The listing builds one solid part. Answer for the finished solid, in the listing's coordinates (mm). Give positions to 0.01 mm unless a question says otherwise; leave off trailing zeros. Write each loop counter-clockwise with the first axis right and the second up, starting at its lowest first coordinate (ties: lowest second). Pieces come first, ordered by that corner, then holes. Notation, with made-up numbers: (-24.75, 16) -> (15.25, 16) arc R20 ccw to (15.25, 21) -> close; hole circle Ø5 at (21, 46.5). An arc over 180 degrees is marked (long way). Put each result on its own line as item: value. Start each with the question number.
1) A cutting plane is placed at D-D (y = -71.5). Write down the section's boundary in (x, z), then the cut area to 3 significant figures.
2) A cutting plane is placed at A-A (z = 3.4). Give the number of separate pieces and of enclosed holes in the cut face, then the cut area to 3 significant figures.
3) Find the intervals of material crossed by line 1 along Y through (x, z) = (75, 1.3); line 2 along X through (y, z) = (-91.5, 3.5); line 3 along Y through (x, z) = (89, 3.25), in increasing order. Write a range as from..to.
4) Flat-ended cylindrical pins translate along their axes: pin 1 Ø1.3 at (y, z) = (-39.5, 1.5) entering from +X; pin 2 Ø1.3 at (x, z) = (155.5, 3.5) entering from +Y. Find the tip coordinate at first contact, or state that the pin passes through.
5) A cutting plane is placed at C-C (x = 32.5). Write down the section's boundary in (y, z).
6) A cutting plane is placed at B-B (y = -50). Write down the section's boundary in (x, z), then the cut area to 3 significant figures.
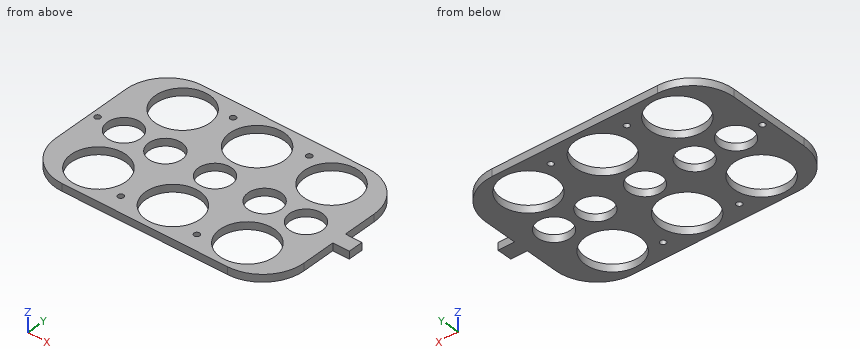
Autodesk Inventor part; units mm, degrees
ref_plane "YZ Plane" through (0, 0, 0) normal (1, 0, 0) x (0, 1, 0)
ref_plane "XZ Plane" through (0, 0, 0) normal (0, 1, 0) x (-1, 0, 0)
ref_plane "XY Plane" through (0, 0, 0) normal (0, 0, 1) x (1, 0, 0)
sketch "Sketch1" plane through (0, 0, 0) normal (0, 0, 1) x (1, 0, 0)
  line L0 (0, 0) -> (150, 0)
  line L1 (150, 0) -> (150, -100)
  line L2 (150, -100) -> (0, -100)
  line L3 (0, -100) -> (0, 0)
  circle A0 centre (30, -20) radius 16.5
  circle A1 centre (30, -80) radius 16.5
  circle A2 centre (75, -20) radius 16.5
  circle A3 centre (120, -20) radius 16.5
  circle A4 centre (75, -80) radius 16.5
  circle A5 centre (120, -80) radius 16.5
  circle A6 centre (20, -50) radius 10
  circle A7 centre (45, -50) radius 10
  circle A8 centre (75, -50) radius 10
  circle A9 centre (105, -50) radius 10
  circle A10 centre (130, -50) radius 10
  circle A11 centre (52, -10) radius 1.75
  circle A12 centre (98, -10) radius 1.75
  circle A13 centre (52, -90) radius 1.75
  circle A14 centre (98, -90) radius 1.75
  circle A15 centre (4, -50) radius 1.75
  dimension "d0" = 150
  dimension "d1" = 100
  dimension "d2" = 33
  dimension "d3" = 33
  dimension "d5" = 33
  dimension "d6" = 33
  dimension "d8" = 33
  dimension "d9" = 33
  dimension "d10" = 20
  dimension "d11" = 20
  dimension "d12" = 20
  dimension "d13" = 30
  dimension "d14" = 30
  dimension "d15" = 75
  dimension "d16" = 30
  dimension "d17" = 75
  dimension "d18" = 30
  dimension "d19" = 20
  dimension "d20" = 20
  dimension "d21" = 20
  dimension "d22" = 20
  dimension "d23" = 20
  dimension "d25" = 20
  dimension "d26" = 20
  dimension "d27" = 20
  dimension "d28" = 20
  dimension "d29" = 20
  dimension "d30" = 25
  dimension "d31" = 25
  dimension "d32" = 50
  dimension "d33" = 50
  dimension "d34" = 50
  dimension "d35" = 50
  dimension "d36" = 50
  dimension "d37" = 75
  dimension "d56" = 3.5
  dimension "d57" = 3.5
  dimension "d58" = 3.5
  dimension "d59" = 3.5
  dimension "d60" = 10
  dimension "d61" = 10
  dimension "d62" = 10
  dimension "d63" = 10
  dimension "d64" = 52
  dimension "d65" = 52
  dimension "d66" = 52
  dimension "d67" = 52
  dimension "d74" = 3.5
  dimension "d75" = 4
  dimension "d76" = 50
extrude "Extrusion5" add sketch "Sketch1" along normal blind 4.5
sketch "Sketch4" plane through (150, -100, 0) normal (1, 0, 0) x (0, 0, -1)
  line L0 (0, 0) -> (-4.5, 0)
  line L1 (0, 100) -> (-4.5, 100)
  line L2 (-4.5, 100) -> (-4.5, 0)
  line L3 (-4.5, 0) -> (0, 0)
  line L4 (0, 0) -> (0, 100)
  line L5 (-4.5, 40) -> (-4.5, 60)
  line L6 (-4.5, 45.5) -> (0, 45.5)
  line L7 (0, 45.5) -> (0, 54.5)
  line L8 (0, 54.5) -> (-4.5, 54.5)
  line L9 (-4.5, 54.5) -> (-4.5, 45.5)
  dimension "d79" = 9
  dimension "d80" = 45.5
extrude "Extrusion6" add sketch "Sketch4" along normal blind 10 contours L6 L2 L8 L4
fillet "Fillet9" radius 25 1 edges at (150, 0, 2.25)
fillet "Fillet10" radius 25 1 edges at (150, -100, 2.25)
fillet "Fillet11" radius 25 1 edges at (0, -100, 2.25)
fillet "Fillet12" radius 25 1 edges at (0, 0, 2.25)
properties part number "Bandeja de tubos"
Reply:
1. outline: (0, 0) -> (15.86, 0) -> (15.86, 4.5) -> (0, 4.5) -> close; (44.14, 0) -> (60.86, 0) -> (60.86, 4.5) -> (44.14, 4.5) -> close; (89.14, 0) -> (105.86, 0) -> (105.86, 4.5) -> (89.14, 4.5) -> close; (134.14, 0) -> (150, 0) -> (150, 4.5) -> (134.14, 4.5) -> close
1. area: 293 mm2
2. separate pieces: 1
2. enclosed holes: 16
2. area: 7,800 mm2
3. line 1: y = -100..-96.5, -63.5..-60, -40..-36.5, -3.5..0
3. line 2: x = 6.22..18.17, 41.83..51.1, 52.9..63.17, 86.83..97.1, 98.9..108.17, 131.83..143.78
3. line 3: y = -100..-88.73, -71.27..-28.73, -11.27..0
4. pin 1: stops at x = 150
4. pin 2: stops at y = -45.5
5. outline: (-100, 0) -> (-96.31, 0) -> (-96.31, 4.5) -> (-100, 4.5) -> close; (-63.69, 0) -> (-36.31, 0) -> (-36.31, 4.5) -> (-63.69, 4.5) -> close; (-3.69, 0) -> (0, 0) -> (0, 4.5) -> (-3.69, 4.5) -> close
6. outline: (0, 0) -> (2.25, 0) -> (2.25, 4.5) -> (0, 4.5) -> close; (5.75, 0) -> (10, 0) -> (10, 4.5) -> (5.75, 4.5) -> close; (30, 0) -> (35, 0) -> (35, 4.5) -> (30, 4.5) -> close; (55, 0) -> (65, 0) -> (65, 4.5) -> (55, 4.5) -> close; (85, 0) -> (95, 0) -> (95, 4.5) -> (85, 4.5) -> close; (115, 0) -> (120, 0) -> (120, 4.5) -> (115, 4.5) -> close; (140, 0) -> (160, 0) -> (160, 4.5) -> (140, 4.5) -> close
6. area: 254 mm2
